Can you work these out from the model? Positions are in its coordinate system, mm. Coordinates: 2 decimals unless noted, no trailing zeros. Loops run counter-clockwise (first coordinate to the right, second up) from the corner with the lowest first, then second, coordinate; pieces in that order, holes last. Notation, with made-up numbers: (33, 58) - (41, 58) arc R19 ccw to (41, 71) - close; hole circle Ø5 at (61.25, 60.5). An arc over 180 degrees is marked (long way). Put each result on its own line as item: value. Start each with the question number.
from build123d import *

# Parameters (mm, degrees)
CROQUIS1_R              = 4.25
SALIENTE_EXTRUIR1_DEPTH = 20
REDONDEO1_R             = 0.5
CROQUIS2_R              = 0.5
SALIENTE_EXTRUIR2_DEPTH = 5


with BuildPart() as part:
    # Croquis1 → Saliente-Extruir1 (new body)
    with BuildSketch(Plane(origin=(0, 0, 0), x_dir=(1, 0, 0), z_dir=(0, 1, 0))):
        with Locations(Location((0, 0, 0), (0, 0, 270))):
            Circle(CROQUIS1_R)
    extrude(amount=SALIENTE_EXTRUIR1_DEPTH)

    # Redondeo1
    redondeo1_edges = [part.edges().sort_by_distance(p)[0] for p in [
        (0, 20, -4.25),
    ]]
    fillet(redondeo1_edges, radius=REDONDEO1_R)

    # Croquis2 → Saliente-Extruir2 (add)
    with BuildSketch(Plane(origin=(0, 20, 0), x_dir=(1, 0, 0), z_dir=(0, 1, 0))):
        with Locations(Location((0, 0, 0), (0, 0, 270))):
            Circle(CROQUIS2_R)
    extrude(amount=SALIENTE_EXTRUIR2_DEPTH)


solid = part.part
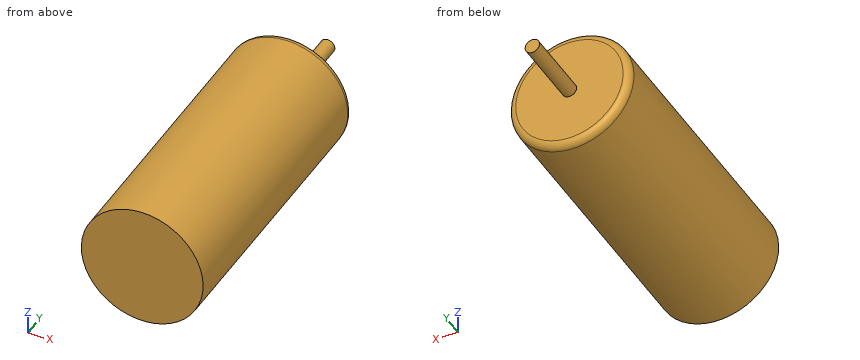
Q1. Please list where these lines run through material, in increasing order: line 1 along Y through (x, z) = (-3, -0.5); line 2 along X through (y, z) = (6.5, 2); line 3 along X through (y, z) = (14.5, 2.25). Write a range as [from, to].
Q2. I want a section at B-B on z = 0. List the corners of the cut face in (x, y) for me, and give its area (3 significant figures).
Q3. I want a section at C-C on y = 11.25. List the corners of the cut face in (x, z) for me, and give its area (3 significant figures).
Q4. Will these pins go through, and if not, where does the flat tip stop? pin 1 (1 mm diameter, centred on x = 1, y = 7, fed in from -Z); pin 2 (5 mm diameter, centred on x = 3, y = 20, fed in from +Z).
Q5. I want a section at A-A on x = 0. List the corners of the cut face in (y, z) for me.
Calculated:
1. line 1: [0, 20]
1. line 2: [-3.75, 3.75]
1. line 3: [-3.61, 3.61]
2. outline: (-4.25, 0) - (4.25, 0) - (4.25, 19.5) arc R0.5 ccw to (3.75, 20) - (0.5, 20) - (0.5, 25) - (-0.5, 25) - (-0.5, 20) - (-3.75, 20) arc R0.5 ccw to (-4.25, 19.5) - close
2. area: 175 mm2
3. outline: circle Ø8.5 at (0, 0)
3. area: 56.7 mm2
4. pin 1: z = -4.22
4. pin 2: z = 4.21
5. outline: (0, -4.25) - (19.5, -4.25) arc R0.5 ccw to (20, -3.75) - (20, -0.5) - (25, -0.5) - (25, 0.5) - (20, 0.5) - (20, 3.75) arc R0.5 ccw to (19.5, 4.25) - (0, 4.25) - close
